Could you check a few things on this model? Use its own coordinates, in mm. Face numbers are marked on the shaded views. A direction names the side the tool comes from. Give positions to 0.01 mm unless a question says otherwise; leave off trailing zeros. Write each loop counter-clockwise with the first axis right and the second up, starting at its lowest first coordinate (ties: lowest second). Pieces come first, ordered by that corner, then holes. Notation, with made-up numbers: M -26.75,61.5 L -21.75,61.5 A25 cw -21.75,78.5 Z; hole C -26.75,-37.5 d4. An arc over 180 degrees is marked long. Use one line per item in the form item = value.
from build123d import *

# Parameters (mm, degrees)
SKETCH1_W           = 60
SKETCH1_H           = 60
BOSS_EXTRUDE1_DEPTH = 5
SKETCH2_R           = 2.75
CUT_EXTRUDE1_DEPTH  = 5
FILLET1_R           = 5
SKETCH3_R           = 16
BOSS_EXTRUDE2_DEPTH = 8
SKETCH4_R           = 7
CUT_EXTRUDE2_DEPTH  = 14


with BuildPart() as part:
    # Sketch1 → Boss-Extrude1 (new body)
    with BuildSketch(Plane.XY):
        Rectangle(SKETCH1_W, SKETCH1_H)
    extrude(amount=BOSS_EXTRUDE1_DEPTH)

    # Sketch2 → Cut-Extrude1 (cut)
    with BuildSketch(Plane.XY.offset(5)):
        with Locations((-25, 25)):
            Circle(SKETCH2_R)
        with Locations((25, 25)):
            Circle(SKETCH2_R)
        with Locations((25, -25)):
            Circle(SKETCH2_R)
        with Locations((-25, -25)):
            Circle(SKETCH2_R)
    extrude(amount=-CUT_EXTRUDE1_DEPTH, mode=Mode.SUBTRACT)

    # Fillet1
    fillet1_edges = [part.edges().sort_by_distance(p)[0] for p in [
        (-30, 30, 2.5),
        (30, 30, 2.5),
        (30, -30, 2.5),
        (-30, -30, 2.5),
    ]]
    fillet(fillet1_edges, radius=FILLET1_R)

    # Sketch3 → Boss-Extrude2 (add)
    with BuildSketch(Plane.XY.offset(5)):
        Circle(SKETCH3_R)
    extrude(amount=BOSS_EXTRUDE2_DEPTH)

    # Sketch4 → Cut-Extrude2 (cut, through all)
    with BuildSketch(Plane.XY.offset(13)):
        Circle(SKETCH4_R)
    extrude(amount=-CUT_EXTRUDE2_DEPTH, mode=Mode.SUBTRACT)


solid = part.part
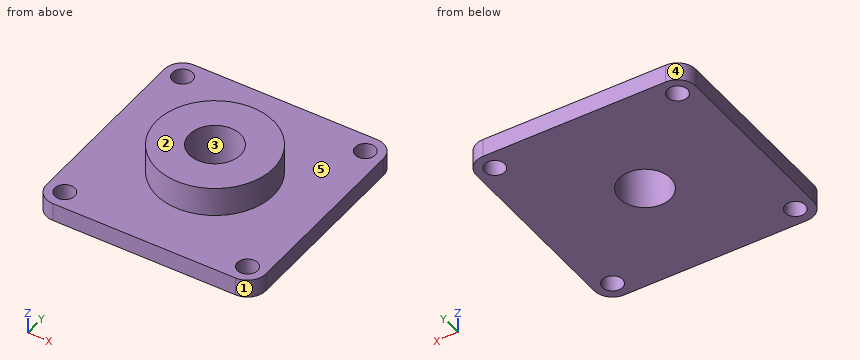
1) I want a section at A-A, the plane x = 0. Please give me the cut outline in (y, z), plus the area to 3 significant figures.
Checked values:
outline = M -30,0 L -7,0 L -7,13 L -16,13 L -16,5 L -30,5 Z; M 7,0 L 30,0 L 30,5 L 16,5 L 16,13 L 7,13 Z
area = 374 mm2
2) For the marked faces 4 and 5, which set-ups out of +Z, -Z, +X, -X, +Y, -Y let a thin tool reach every point of the face, with its end or its side?
Checked values:
face_4 = +Z, -Z, -X, +Y
face_5 = +Z
3) Thinking about a two-plate mould opening in Y: for the marked faces 1, 2 and 3, which applies, released by +Y, released by -Y, zero draft, split by the parting line, or undercut?
Checked values:
face_1 = released by -Y
face_2 = zero draft
face_3 = undercut
4) If I drill on L1, parallel to Y at x = -25, z = 3.7; L2, parallel to Z at x = 2, y = -21.5; L3, parallel to X at y = 3, z = 8.5, over which ranges is the centre line in solid material (lowest first)?
Checked values:
L1 = -30 to -27.75, -22.25 to 22.25, 27.75 to 30
L2 = 0 to 5
L3 = -15.72 to -6.32, 6.32 to 15.72
5) I want a section at D-D, the plane z = 11.5. Please give me the cut outline in (x, y).
Checked values:
outline = C 0,0 d32; hole C 0,0 d14
6) I want a section at C-C, the plane z = 2. Please give me the cut outline in (x, y).
Checked values:
outline = M -30,-25 A5 ccw -25,-30 L 25,-30 A5 ccw 30,-25 L 30,25 A5 ccw 25,30 L -25,30 A5 ccw -30,25 Z; hole C -25,-25 d5.5; hole C -25,25 d5.5; hole C 0,0 d14; hole C 25,-25 d5.5; hole C 25,25 d5.5
7) For pin 1 Ø5 at (x, y) = (25, 25) entering from +Z; pin 2 Ø5 at (x, y) = (-22.5, 19) entering from -Z; pin 3 Ø1.5 at (y, z) = (0, 6.5) entering from +X; pin 4 Ø9 at (x, y) = (-25, -25) entering from +Z, each with a flat end and sliding along its axis, tell me the tip position at first contact or that it passes through.
Checked values:
pin_1 = through
pin_2 = 0
pin_3 = 16
pin_4 = 5
